Build history of the part. All positions in model axes, mm. A direction names the side the tool comes from. Give positions to 0.01 mm unless a question says otherwise; leave off trailing zeros. Write each loop counter-clockwise with the first axis right and the second up, starting at its lowest first coordinate (ties: lowest second). Pieces come first, ordered by that corner, then holes. Notation, with made-up numbers: M 75,12 L 134,12 A15 ccw 134,39 Z; hole C -29,39 d11. An arc over 180 degrees is marked long. One line per item, written item: value. Start each with the question number.
from build123d import *

# Parameters (mm, degrees)
SKETCH2_R           = 3.048
BOSS_EXTRUDE1_DEPTH = 17.272
SKETCH3_W           = 17.78
SKETCH3_H           = 5.08
BOSS_EXTRUDE2_DEPTH = 5.08
SKETCH4_R           = 2.54
BOSS_EXTRUDE3_DEPTH = 6.35
BOSS_EXTRUDE4_DEPTH = 6.35


with BuildPart() as part:
    # Sketch2 → Boss-Extrude1 (new body)
    with BuildSketch(Plane.XY):
        Circle(SKETCH2_R)
    extrude(amount=BOSS_EXTRUDE1_DEPTH)

    # Sketch3 → Boss-Extrude2 (add)
    with BuildSketch(Plane.XY.offset(17.272)):
        Rectangle(SKETCH3_W, SKETCH3_H)
    extrude(amount=BOSS_EXTRUDE2_DEPTH)

    # Sketch4 → Boss-Extrude3 (add)
    with BuildSketch(Plane.XY.offset(22.352)):
        with Locations(Location((0, 0, 0), (0, 0, 270))):
            Circle(SKETCH4_R)
    extrude(amount=BOSS_EXTRUDE3_DEPTH)

    # Sketch5 → Boss-Extrude4 (add)
    with BuildSketch(Plane.XY.offset(28.702)):
        Polygon((-3.175, 3.175), (-3.175, 9.525), (3.175, 9.525), (3.175, 3.175), (9.525, 3.175), (9.525, -3.175), (3.175, -3.175), (3.175, -9.525), (-3.175, -9.525), (-3.175, -3.175), (-9.525, -3.175), (-9.525, 3.175), align=None)
    extrude(amount=BOSS_EXTRUDE4_DEPTH)


solid = part.part
1) Probe line 1 along Z through (x, y) = (-3.5, -0.5); line 2 along Z through (x, y) = (-1, 2.5); line 3 along Z through (x, y) = (-3.25, -3). List the from-to ranges inside material, lowest first. Write a range as from..to.
2) Tool access for faces 5 (the face through (-0.4, 3.02, 8.52)), 6 (the face through (6, -3.175, 32)), 7 (the face through (-3.175, 6, 32)), 8 (the face through (-8.89, 0, 20)), 9 (the face through (6, 3.175, 32)): list every direction of +Z, -Z, +X, -X, +Y, -Y with a clear straight run to the whole face (end or side of a thin tool).
3) Band-saw the part on B-B (y = 0). List the corners of the cut face in (x, z) (3 decimals).
4) Band-saw the part on A-A (x = -7). List the corners of the cut face in (y, z) (3 decimals).
5) Band-saw the part on D-D (z = 3.5). List the corners of the cut face in (x, y).
6) Mould opens along Z. For faces 1 (the face through (-6, -3.175, 32)), 2 (the face through (-6, 0, 17.272)), 3 (the face through (2.52, 0.33, 25.48)), 4 (the face through (-2, 2, 28.702)) say: released by +Z, released by -Z, zero draft, split by the parting line, or undercut.
7) Drop flat-ended pins along their axis: P1, Ø8, axis at y = -1, z = 8, coming from the -X side; P2, Ø3, axis at y = 5.5, z = 31, coming from the +X side (3 decimals); P3, Ø5, axis at x = 7.5, z = 33.5, coming from the +Y side (3 decimals). Give the stop position or say it passes through.
8) Band-saw the part on C-C (z = 27). List the corners of the cut face in (x, y), then the cut area to 3 significant figures.
Model answer:
1. line 1: z = 17.27..22.35, 28.7..35.05
1. line 2: z = 0..22.35, 28.7..35.05
1. line 3: z = 28.7..35.05
2. face 5: -Z
2. face 6: +Z, -Z, +X, -Y
2. face 7: +Z, -Z, -X, +Y
2. face 8: -Z, -X, +Y, -Y
2. face 9: +Z, -Z, +X, +Y
3. outline: M -9.525,28.702 L -2.54,28.702 L -2.54,22.352 L -8.89,22.352 L -8.89,17.272 L -3.048,17.272 L -3.048,0 L 3.048,0 L 3.048,17.272 L 8.89,17.272 L 8.89,22.352 L 2.54,22.352 L 2.54,28.702 L 9.525,28.702 L 9.525,35.052 L -9.525,35.052 Z
4. outline: M -3.175,28.702 L 3.175,28.702 L 3.175,35.052 L -3.175,35.052 Z; M -2.54,17.272 L 2.54,17.272 L 2.54,22.352 L -2.54,22.352 Z
5. outline: C 0,0 d6.1
6. face 1: zero draft
6. face 2: released by -Z
6. face 3: undercut
6. face 4: undercut
7. P1: stops at x = -3.05
7. P2: stops at x = 3.175
7. P3: stops at y = 3.175
8. outline: C 0,0 d5.08
8. area: 20.3 mm²
